Check sheet for the modelled part. Datum: model origin and axes. Units: mm. A direction names the side the tool comes from. Give positions to 0.01 mm unless a question says otherwise; leave off trailing zeros. Write each loop counter-clockwise with the first axis right and the second up, starting at its lowest first coordinate (ties: lowest second). Pieces come first, ordered by that corner, then holes. Notation, with made-up numbers: M -7.75,58 L 13.25,58 A17 cw 13.25,89 Z; hole C 38.5,37 d4. An arc over 180 degrees is marked long. Write item = value, one per line. Start each with the question number.
1) Set-up check for faces 1 (the face through (-74.373, -47.545, 25.865)), 2 (the face through (1, -36.512, -1)), 3 (the face through (1.245, -36.357, 25.312)), 4 (the face through (1, 47, 25.082)): record each of +Z, -Z, +X, -X, +Y, -Y from which the full face is reachable in a straight line by a thin tool's end or side.
2) Draft check along Y on faces 5 (the face through (-11.25, 46.51, 25.87)), 6 (the face through (1.24, -35.08, -26.9)), 7 (the face through (74.511, 46.925, 25.865)), 8 (the face through (1, 0, -28.258)). Enter one of: pulls with the +Y half, pulls with the -Y half, needs draft (parallel to the pull), parting line crosses it, or undercut.
3) Sectioned sample at A-A, the plane x = -57.15. Count the separate pieces of the cut face and the enclosed holes in it, then the cut area to 3 significant figures.
4) Scan lines: L1, parallel to Y at x = -34.5, z = 9.5 (1 decimal); L2, parallel to Y at x = 76.2, z = 26.25 (3 decimals); L3, parallel to Z at x = 26, y = -20.5. Record each from-to range of solid material in increasing order.
5) Gauge pin test, flat ends, axial feed: pin 1 (22.5 mm diameter, centred on x = -5.5, z = -3, fed in from -Y); pin 2 (5 mm diameter, centred on y = 29, z = -22.5, fed in from +X); pin 3 (6 mm diameter, centred on x = 76.2, y = -47.625, fed in from -Z); pin 4 (2 mm diameter, centred on x = 51.5, y = -12, fed in from +Z). Record the tip position at first contact, or that the pin passes through.
6) Sectioned sample at B-B, the plane z = -5. Record the cut outline in (x, y) (1 decimal).
from build123d import *

# Parameters (mm, degrees)
BASE_FLANGE1_DEPTH          = 88.9
F_27_0_144_DIAMETER_HOLE1_D = 3.6576
F_1_4_0_25_DIAMETER_HOLE1_D = 6.35


# Sheet-metal steps are written as plain solids
with BuildPart() as part:
    # Sketch1 → Base-Flange1 (new, symmetric)
    with BuildSketch(Plane.YZ):
        with BuildLine():
            Line((-53.975, 26.67), (-39.6875, 26.67))
            ThreePointArc((-39.6875, 26.67), (-36.319903955, 25.275096045), (-34.925, 21.9075))
            Line((-34.925, 21.9075), (-34.925, -23.495))
            ThreePointArc((-34.925, -23.495), (-33.99506403, -25.74006403), (-31.75, -26.67))
            Line((-31.75, -26.67), (31.75, -26.67))
            ThreePointArc((31.75, -26.67), (33.99506403, -25.74006403), (34.925, -23.495))
            Line((34.925, -23.495), (34.925, 21.9075))
            ThreePointArc((34.925, 21.9075), (36.319903955, 25.275096045), (39.6875, 26.67))
            Line((39.6875, 26.67), (53.975, 26.67))
            Line((53.975, 26.67), (53.975, 25.0825))
            Line((53.975, 25.0825), (39.6875, 25.0825))
            ThreePointArc((39.6875, 25.0825), (37.44243597, 24.15256403), (36.5125, 21.9075))
            Line((36.5125, 21.9075), (36.5125, -23.495))
            ThreePointArc((36.5125, -23.495), (35.117596045, -26.862596045), (31.75, -28.2575))
            Line((31.75, -28.2575), (-31.75, -28.2575))
            ThreePointArc((-31.75, -28.2575), (-35.117596045, -26.862596045), (-36.5125, -23.495))
            Line((-36.5125, -23.495), (-36.5125, 21.9075))
            ThreePointArc((-36.5125, 21.9075), (-37.44243597, 24.15256403), (-39.6875, 25.0825))
            Line((-39.6875, 25.0825), (-53.975, 25.0825))
            Line((-53.975, 25.0825), (-53.975, 26.67))
        make_face()
    extrude(amount=BASE_FLANGE1_DEPTH, both=True)

    # #27 (0.144) Diameter Hole1 (through all)
    with Locations(Plane.XY.offset(26.67)):
        with Locations((-76.2, 47.625), (-12.7, 47.625), (76.2, 47.625), (76.2, -47.625), (-12.7, -47.625), (-76.2, -47.625)):
            Hole(F_27_0_144_DIAMETER_HOLE1_D / 2)

    # 1/4 (0.25) Diameter Hole1 (through all)
    with Locations(Plane.XZ.offset(36.5125)):
        with Locations((-57.15, 16.1925)):
            Hole(F_1_4_0_25_DIAMETER_HOLE1_D / 2)


solid = part.part
Data:
q1.face_1 = +Z, -Z
q1.face_2 = -Z, +X, -X, -Y
q1.face_3 = +Z, +X, -X
q1.face_4 = -Z, +X, -X, +Y
q2.face_5 = undercut
q2.face_6 = pulls with the -Y half
q2.face_7 = undercut
q2.face_8 = needs draft
q3.separate_pieces = 3
q3.enclosed_holes = 0
q3.area = 310 mm2
q4.L1 = -36.5 to -34.9, 34.9 to 36.5
q4.L2 = -53.975 to -49.454, -45.796 to -37.732, 37.732 to 45.796, 49.454 to 53.975
q4.L3 = -28.26 to -26.67
q5.pin_1 = -36.51
q5.pin_2 = through
q5.pin_3 = 25.08
q5.pin_4 = -26.67
q6.outline = M -88.9,-36.5 L 88.9,-36.5 L 88.9,-34.9 L -88.9,-34.9 Z; M -88.9,34.9 L 88.9,34.9 L 88.9,36.5 L -88.9,36.5 Z
